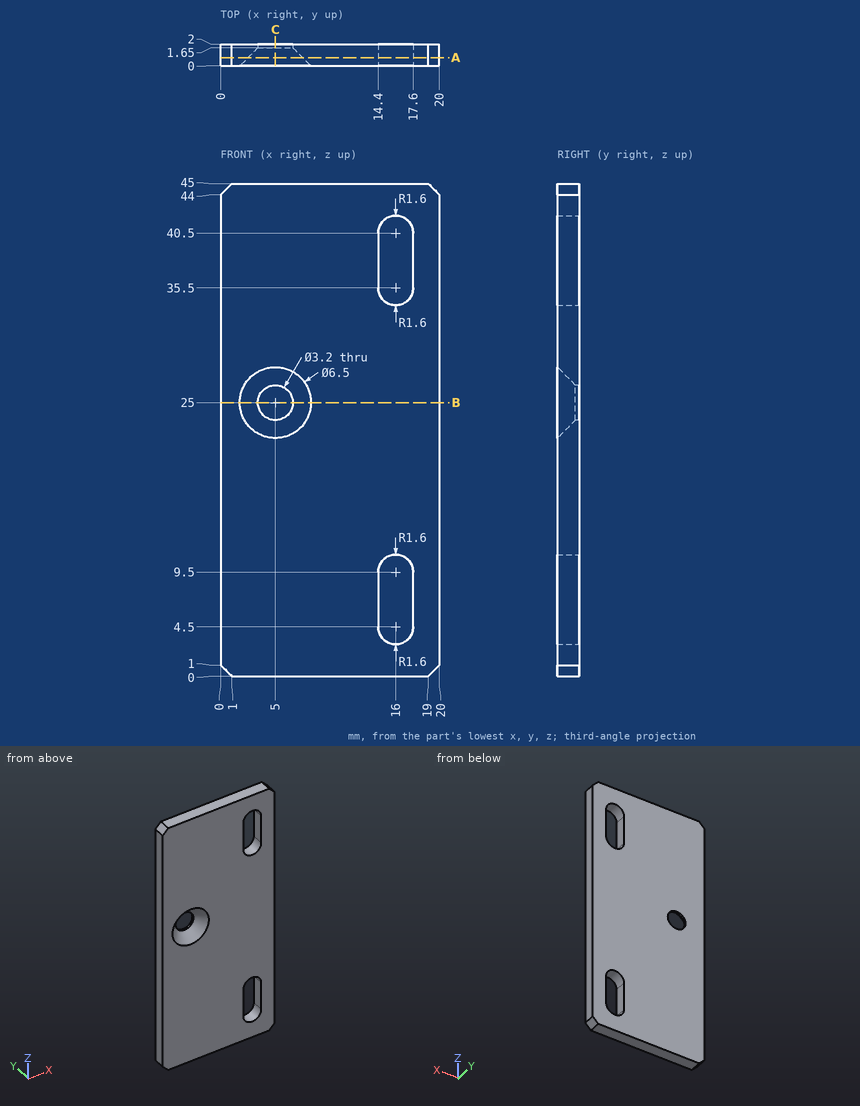
Can you work these out from the drawing? Everything is in mm from the part's minimum corner. Round coordinates to 2 decimals unless told otherwise and drop trailing zeros. Loops run counter-clockwise (first coordinate to the right, second up) from the corner with the lowest first, then second, coordinate; pieces in that order, holes last. Notation, with made-up numbers: (62.25, 22) - (117.25, 22) arc R32 ccw to (117.25, 54) - close; hole circle Ø2 at (-4.75, 80.5). An arc over 180 degrees is marked (long way). Answer in a Markdown table with one row per item. Add a question column.
Q1. I want a section at A-A on y = 0.75. List the corners of the cut face in (x, z) for me, and give its area (3 significant figures).
Q2. For pin 1 Ø4 at (x, z) = (5, 25) entering from -Y; pin 2 Ø1 at (y, z) = (1, 8) entering from -X, each with a flat end and sliding along its axis, tell me the tip position at first contact or that it passes through.
Q3. I need wall thicknesses on L1, parallel to X at y = 1.15, z = 38.5; L2, parallel to Z at x = 5, y = 1.8; L3, parallel to X at y = 1.85, z = 25. Which ranges of each line are inside material? Lowest first, please.
Q4. I want a section at B-B on z = 25. List the corners of the cut face in (x, y) for me.
Q5. I want a section at C-C on x = 5. List the corners of the cut face in (y, z) for me.
A:
| question | item | result |
|---|---|---|
| 1 | outline | (0, 1) - (1, 0) - (19, 0) - (20, 1) - (20, 44) - (19, 45) - (1, 45) - (0, 44) - close; hole circle Ø5 at (5, 25); hole (14.4, 4.5) arc R1.6 ccw to (17.6, 4.5) - (17.6, 9.5) arc R1.6 ccw to (14.4, 9.5) - close; hole (14.4, 35.5) arc R1.6 ccw to (17.6, 35.5) - (17.6, 40.5) arc R1.6 ccw to (14.4, 40.5) - close |
| 1 | area | 830 mm^2 |
| 2 | pin 1 | y = 1.25 |
| 2 | pin 2 | x = 0 |
| 3 | L1 | 0 to 14.4, 17.6 to 20 |
| 3 | L2 | 0 to 23.4, 26.6 to 45 |
| 3 | L3 | 0 to 3.4, 6.6 to 20 |
| 4 | outline | (0, 0) - (1.75, 0) - (3.4, 1.65) - (3.4, 2) - (0, 2) - close; (6.6, 1.65) - (8.25, 0) - (20, 0) - (20, 2) - (6.6, 2) - close |
| 5 | outline | (0, 0) - (2, 0) - (2, 23.4) - (1.65, 23.4) - (0, 21.75) - close; (0, 28.25) - (1.65, 26.6) - (2, 26.6) - (2, 45) - (0, 45) - close |
